Job drawing, mm, ordinate dimensions from the low corner. One solid piece. Give positions to 0.01 mm unless a question says otherwise; leave off trailing zeros. Loops run counter-clockwise (first coordinate to the right, second up) from the corner with the lowest first, then second, coordinate; pieces in that order, holes last. Notation, with made-up numbers: (-9.5, 7) -> (0.5, 7) arc R30 cw to (0.5, 36) -> close; hole circle Ø11 at (78, 20). An arc over 180 degrees is marked (long way). Answer as a JSON object with one key per item and string values. Group by question number.
Q1. Band-saw the part on B-B, the plane x = 96.5. Write the cut outline in (y, z).
Q2. Two-plate mould, pull along X, no slides. Class the marked faces 1, 2 and 3: pulls with the +X half, pulls with the -X half, needs draft (parallel to the pull), parting line crosses it, or undercut.
Q3. Band-saw the part on A-A, the plane z = 49. Write the cut outline in (x, y) (1 decimal), plus the area to 3 significant figures.
Q4. Band-saw the part on C-C, the plane y = 23. Write the cut outline in (x, z) (1 decimal).
Q5. Band-saw the part on D-D, the plane x = 139. Write the cut outline in (y, z).
Q6. Wall check: probe 1 along X at (y, z) = (18.5, 7.5) (1 decimal); probe 2 along Y at (x, z) = (96, 2); probe 3 along Z at (x, y) = (126.5, 15). Give the ranges that are in metal, low to high. Write a range as from..to.
Q7. Drop flat-ended pins along their axis: pin 1 (20 mm diameter, centred on x = 95.5, y = 18.5, fed in from +Z); pin 2 (18 mm diameter, centred on x = 96.5, y = 20, fed in from +Z); pin 3 (12 mm diameter, centred on y = 28.5, z = 24.5, fed in from -X); pin 4 (3 mm diameter, centred on y = 8, z = 50, fed in from +X). Give the stop position or say it passes through.
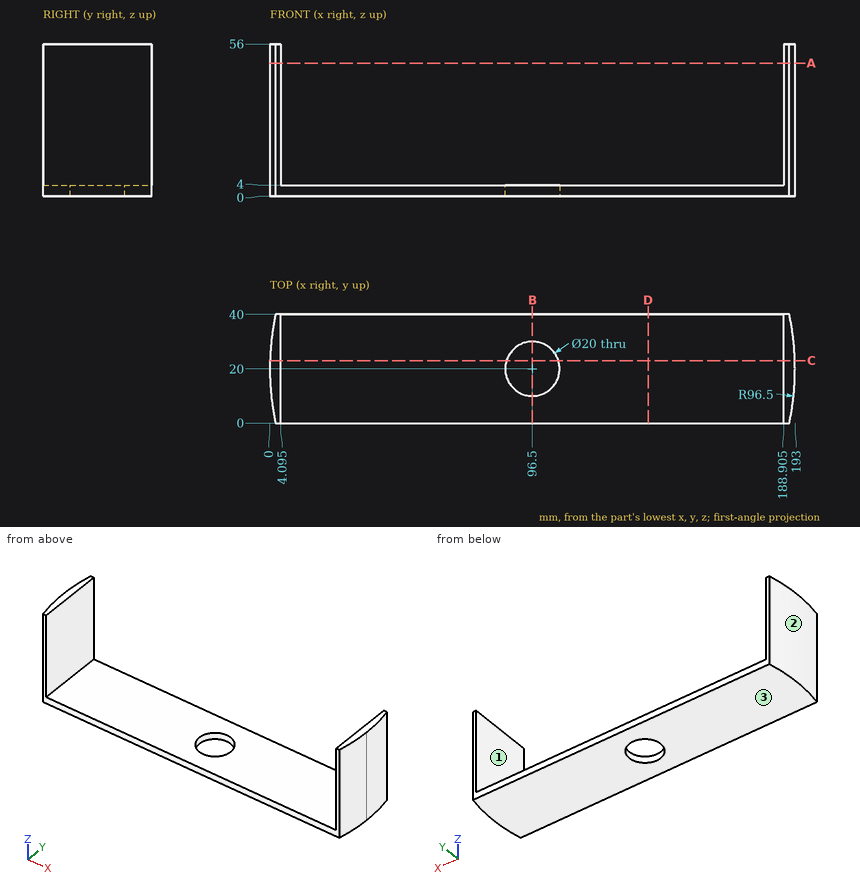
Worked answers:
{
 "1": {"outline": "(0, 0) -> (10, 0) -> (10, 4) -> (0, 4) -> close; (30, 0) -> (40, 0) -> (40, 4) -> (30, 4) -> close"},
 "2": {"face 1": "undercut", "face 2": "pulls with the -X half", "face 3": "needs draft"},
 "3": {"outline": "(2.1, 0) -> (4.1, 0) -> (4.1, 40) -> (2.1, 40) arc R96.5 ccw to start; (188.9, 0) -> (190.9, 0) arc R96.5 ccw to (193, 20) arc R96.5 ccw to (190.9, 40) -> (188.9, 40) -> close", "area": "272 mm2"},
 "4": {"outline": "(0, 0) -> (87, 0) -> (87, 4) -> (4.1, 4) -> (4.1, 56) -> (0, 56) -> close; (106, 0) -> (193, 0) -> (193, 56) -> (188.9, 56) -> (188.9, 4) -> (106, 4) -> close"},
 "5": {"outline": "(0, 0) -> (40, 0) -> (40, 4) -> (0, 4) -> close"},
 "6": {"probe 1": "0..4.1, 188.9..193", "probe 2": "0..10.01, 29.99..40", "probe 3": "0..4"},
 "7": {"pin 1": "z = 4", "pin 2": "through", "pin 3": "x = 0.03", "pin 4": "x = 192.43"}
}
